Input: dimensioned drawing with shaded views. Units: mm. Origin: part minimum x, y, z. A direction names the side the tool comes from. Round coordinates to 2 decimals unless told otherwise and drop trailing zeros. Loops run counter-clockwise (first coordinate to the right, second up) from the corner with the lowest first, then second, coordinate; pieces in that order, holes last. Notation, with made-up numbers: (-14, -5.5) - (41, -5.5) arc R18 cw to (41, 20.5) - close; hole circle Ø7 at (1.5, 57.25). An arc over 180 degrees is marked (long way). One line per question, with ' | ' between items. Start each with the question number.
1. Cut plane D-D (x = 6). Return loops of the section in (y, z).
2. Cut plane C-C (z = 0.35). Return loops of the section in (x, y) (1 decimal), then the cut area to 3 significant figures.
3. Cut plane B-B (x = 18). Return loops of the section in (y, z).
4. Access query for the marked faces 1 and 2. Directions: +Z, -Z, +X, -X, +Y, -Y. A direction counts if a zero-diameter tool reaches every point of the face in a straight line with its end or side. Return the directions, or none.
5. Pin query (flat end, axial travel): pin 1 (0.9 mm diameter, centred on x = 14, y = 4.5, fed in from -Z); pin 2 (0.9 mm diameter, centred on y = 4.5, z = 1, fed in from -X). Return the tip coordinate at first contact, or that it passes through.
6. Cut plane A-A (y = 4.5). Return loops of the section in (x, z).
7. Ray query, line 1 (Y direction, x = 2.5, z = 1.1); line 2 (Y direction, x = 18, z = 2.85); line 3 (X direction, y = 5.25, z = 0.5). Return the intervals inside material, ascending.
8. Mould query, pull axis Y, two halves, no side actions, for the marked faces 3, 4 and 5. Classes: pulls with the +Y half, pulls with the -Y half, needs draft (parallel to the pull), parting line crosses it, or undercut.
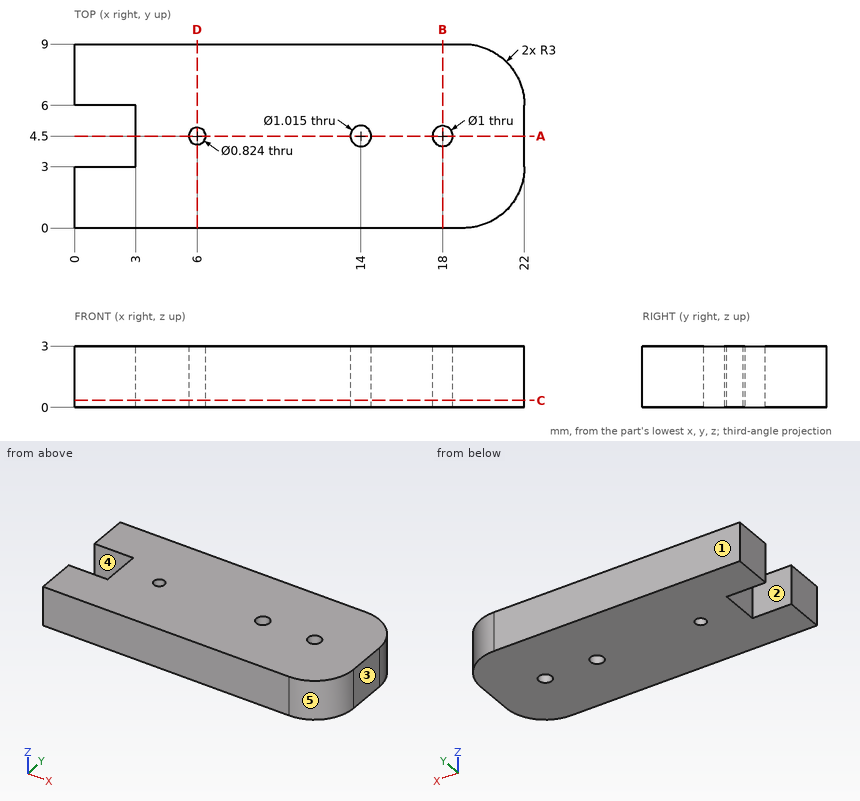
Answers follow:
1) outline: (0, 0) - (4.09, 0) - (4.09, 3) - (0, 3) - close; (4.91, 0) - (9, 0) - (9, 3) - (4.91, 3) - close
2) outline: (0, 0) - (19, 0) arc R3 ccw to (22, 3) - (22, 6) arc R3 ccw to (19, 9) - (0, 9) - (0, 6) - (3, 6) - (3, 3) - (0, 3) - close; hole circle Ø0.8 at (6, 4.5); hole circle Ø1 at (14, 4.5); hole circle Ø1 at (18, 4.5) | area: 183 mm2
3) outline: (0, 0) - (4, 0) - (4, 3) - (0, 3) - close; (5, 0) - (9, 0) - (9, 3) - (5, 3) - close
4) face 1: +Z, -Z, +X, -X, +Y | face 2: +Z, -Z, -X
5) pin 1: passes through | pin 2: stops at x = 3
6) outline: (3, 0) - (5.59, 0) - (5.59, 3) - (3, 3) - close; (6.41, 0) - (13.49, 0) - (13.49, 3) - (6.41, 3) - close; (14.51, 0) - (17.5, 0) - (17.5, 3) - (14.51, 3) - close; (18.5, 0) - (22, 0) - (22, 3) - (18.5, 3) - close
7) line 1: y = 0 to 3, 6 to 9 | line 2: y = 0 to 4, 5 to 9 | line 3: x = 3 to 22
8) face 3: needs draft | face 4: undercut | face 5: pulls with the -Y half
